Verification items for the finished model (mm, model axes). A direction names the side the tool comes from. Give positions to 0.01 mm unless a question says otherwise; leave off trailing zeros. Write each loop counter-clockwise with the first axis right and the second up, starting at its lowest first coordinate (ties: lowest second). Pieces come first, ordered by that corner, then holes. Notation, with made-up numbers: M 64,55.25 L 113,55.25 A17 cw 113,83.25 Z; hole C -13.75,47.5 d3. An arc over 180 degrees is marked long. Answer as a JSON object with one key per item and string values.
```python
from build123d import *

# Parameters (mm, degrees)
F0_W     = 3.3
F0_H     = 15.1
F0_R     = 1.6
F0_W_2   = 10
F0_H_2   = 50
F0_R_2   = 1.1
F1_DEPTH = 3.2


with BuildPart() as f1:
    # F0 (on Front) → F1 (new body)
    with BuildSketch(Plane.XZ):
        with BuildLine():
            Line((17.108108, 110), (-2.891892, 110))
            ThreePointArc((-2.891892, 110), (-11.377174, 106.485281), (-14.891892, 98))
            Line((-14.891892, 98), (-14.891892, 18))
            ThreePointArc((-14.891892, 18), (-9.619814, 5.272078), (3.108108, 0))
            Line((3.108108, 0), (11.108108, 0))
            ThreePointArc((11.108108, 0), (23.83603, 5.272078), (29.108108, 18))
            Line((29.108108, 18), (29.108108, 98))
            ThreePointArc((29.108108, 98), (25.593389, 106.485281), (17.108108, 110))
        make_face()
        with Locations((-8.241892, 40.5)):
            Rectangle(F0_W, F0_H, mode=Mode.SUBTRACT)
        with Locations((7.108108, 11.6)):
            Circle(F0_R, mode=Mode.SUBTRACT)
        with Locations((-8.241892, 75.5)):
            Rectangle(F0_W, F0_H, mode=Mode.SUBTRACT)
        with Locations((16.108108, 55)):
            Rectangle(F0_W_2, F0_H_2, mode=Mode.SUBTRACT)
        with Locations((23.555327, 88.906578)):
            Circle(F0_R_2, mode=Mode.SUBTRACT)
    extrude(amount=F1_DEPTH)


solid = f1.part
```
1) Section check A-A on z = 36. Record the boundary of the cut face in (x, y).
Completed:
{"outline": "M -14.89,-3.2 L -9.89,-3.2 L -9.89,0 L -14.89,0 Z; M -6.59,-3.2 L 11.11,-3.2 L 11.11,0 L -6.59,0 Z; M 21.11,-3.2 L 29.11,-3.2 L 29.11,0 L 21.11,0 Z"}
2) Section check C-C on x = -8.5. Record the boundary of the cut face in (y, z).
Completed:
{"outline": "M -3.2,4.24 L 0,4.24 L 0,32.95 L -3.2,32.95 Z; M -3.2,48.05 L 0,48.05 L 0,67.95 L -3.2,67.95 Z; M -3.2,83.05 L 0,83.05 L 0,108.61 L -3.2,108.61 Z"}
3) Release check for a two-part mould opening along X. For faces 3 (the face through (-9.892, -2, 75)), 4 (the face through (-11.28, -1.58, 106.58)), 5 (the face through (25.69, -1.58, 106.39)) record: pulls with the +X half, pulls with the -X half, needs draft (parallel to the pull), parting line crosses it, or undercut.
Completed:
{"face 3": "undercut", "face 4": "pulls with the -X half", "face 5": "pulls with the +X half"}
4) Access from +Z, -Z, +X, -X, +Y, -Y to the whole of each face (thin tool, end or side, straight path). Record for faces 1 (the face through (7, -2, 110)), 2 (the face through (16, -2, 80)).
Completed:
{"face 1": "+Z, +X, -X, +Y, -Y", "face 2": "+Y, -Y"}
5) Section check B-B on z = 49.5. Record the boundary of the cut face in (x, y).
Completed:
{"outline": "M -14.89,-3.2 L 11.11,-3.2 L 11.11,0 L -14.89,0 Z; M 21.11,-3.2 L 29.11,-3.2 L 29.11,0 L 21.11,0 Z"}
6) Section check D-D on y = -2.5. Record the boundary of the cut face in (x, z), and give its area (3 significant figures).
Completed:
{"outline": "M -14.89,18 A18 ccw 3.11,0 L 11.11,0 A18 ccw 29.11,18 L 29.11,98 A12 ccw 17.11,110 L -2.89,110 A12 ccw -14.89,98 Z; hole M -9.89,32.95 L -6.59,32.95 L -6.59,48.05 L -9.89,48.05 Z; hole M -9.89,67.95 L -6.59,67.95 L -6.59,83.05 L -9.89,83.05 Z; hole C 7.11,11.6 d3.2; hole M 11.11,30 L 21.11,30 L 21.11,80 L 11.11,80 Z; hole C 23.56,88.91 d2.2", "area": "4,030 mm2"}
7) Go/stop test with flat-tipped pins: pin 1 (1.6 mm diameter, centred on x = -7.5, y = -2, fed in from +Z); pin 2 (12 mm diameter, centred on x = -8, z = 42, fed in from -Y); pin 3 (1.5 mm diameter, centred on x = 2, y = -0.5, fed in from -Z); pin 4 (1.6 mm diameter, centred on x = -7.5, y = -1, fed in from -Z). Record where each tip stops, or that it passes through.
Completed:
{"pin 1": "stops at z = 109.38", "pin 2": "stops at y = -3.2", "pin 3": "stops at z = 0", "pin 4": "stops at z = 2.91"}
8) Thickness scan on L1, parallel to X at y = -1.35, z = 48; L2, parallel to X at y = -1.65, z = 82; L3, parallel to Z at x = -7, y = -0.9. Record the ranges inside material, lowest first.
Completed:
{"L1": "x = -14.89 to -9.89, -6.59 to 11.11, 21.11 to 29.11", "L2": "x = -14.89 to -9.89, -6.59 to 29.11", "L3": "z = 3.11 to 32.95, 48.05 to 67.95, 83.05 to 109.27"}
